```python
from build123d import *

# Parameters (mm, degrees)
SKETCH_1_R      = 11
EXTRUDE_1_DEPTH = 4
CHAMFER_1_SIZE  = 0.5


with BuildPart() as part:
    # 草图1 → 拉伸1 (new body)
    with BuildSketch(Plane.XY):
        Circle(SKETCH_1_R)
    extrude(amount=EXTRUDE_1_DEPTH)

    # 倒角1
    chamfer_1_edges = [part.edges().sort_by_distance(p)[0] for p in [
        (-11, 0, 0),
        (-11, 0, 4),
    ]]
    chamfer(chamfer_1_edges, length=CHAMFER_1_SIZE)

    # 草图2 → 打孔尺寸根据十字槽沉头木螺钉的类型1 (revolve, cut)
    with BuildSketch(Plane.YZ):
        Polygon((0, 0), (0, 4), (2.75, 4), (2.75, 2.85), (5.6, 0), align=None)
    revolve(axis=Axis((0, 0, -6.35), (0, 0, 1)), mode=Mode.SUBTRACT)


solid = part.part
```
Input: part model. Units: mm. Frame: model coordinates. Give positions to 0.01 mm unless a question says otherwise; leave off trailing zeros. Order: outer loops, then holes, each group sorted by start corner. A loop starts at its lowest first (then second) coordinate and runs counter-clockwise, first axis right, second up.
1. Material intervals for L1, parallel to Y at x = 0, z = 3.45; L2, parallel to X at y = -0.25, z = 3.7; L3, parallel to Y at x = 0.25, z = 2.6, sorted ascending.
Derived:
L1: y = -11 to -2.75, 2.75 to 11
L2: x = -10.8 to -2.74, 2.74 to 10.8
L3: y = -11 to -2.99, 2.99 to 11
2. Section A-A on y = 0. Return the cut outline in (x, z).
Derived:
outline: (-11, 0.5) - (-10.5, 0) - (-5.6, 0) - (-2.75, 2.85) - (-2.75, 4) - (-10.5, 4) - (-11, 3.5) - close; (2.75, 2.85) - (5.6, 0) - (10.5, 0) - (11, 0.5) - (11, 3.5) - (10.5, 4) - (2.75, 4) - close
3. Pin query (flat end, axial travel): pin 1 (2 mm diameter, centred on y = -2, z = 2.5, fed in from +X); pin 2 (1 mm diameter, centred on x = -3.5, z = 3, fed in from +Y). Return the tip coordinate at first contact, or that it passes through.
Derived:
pin 1: stops at x = 10.95
pin 2: stops at y = 10.58
4. Section C-C on z = 1.7. Return the cut outline in (x, y).
Derived:
outline: circle Ø22 at (0, 0); hole circle Ø7.8 at (0, 0)
